from build123d import *

# Parameters (mm, degrees)
SKETCH1_R           = 8.5
BOSS_EXTRUDE1_DEPTH = 1
SKETCH2_W           = 31
SKETCH2_H           = 23.6
BOSS_EXTRUDE2_DEPTH = 4
SKETCH3_W           = 10
SKETCH3_H           = 23.6
BOSS_EXTRUDE3_DEPTH = 6
SKETCH4_R           = 3.5
BOSS_EXTRUDE4_DEPTH = 1
SKETCH5_R           = 2.5
BOSS_EXTRUDE5_DEPTH = 20.25
SKETCH7_R           = 2.25
CUT_EXTRUDE1_DEPTH  = 12
SKETCH8_R           = 2.25
CUT_EXTRUDE2_DEPTH  = 50.945194964
CHAMFER1_SIZE       = 0.5


with BuildPart() as part:
    # Sketch1 → Boss-Extrude1 (new body)
    with BuildSketch(Plane.XY):
        with Locations((15.5, 11.8)):
            Circle(SKETCH1_R)
    extrude(amount=BOSS_EXTRUDE1_DEPTH)

    # Sketch2 → Boss-Extrude2 (add)
    with BuildSketch(Plane.XY.offset(1)):
        with Locations((15.5, 11.8)):
            Rectangle(SKETCH2_W, SKETCH2_H)
    extrude(amount=BOSS_EXTRUDE2_DEPTH)

    # Sketch3 → Boss-Extrude3 (add)
    with BuildSketch(Plane.XY.offset(5)):
        with Locations((15.5, 11.8)):
            Rectangle(SKETCH3_W, SKETCH3_H)
    extrude(amount=BOSS_EXTRUDE3_DEPTH)

    # Sketch4 → Boss-Extrude4 (add)
    with BuildSketch(Plane.XY.offset(11)):
        with Locations((15.5, 11.8)):
            Circle(SKETCH4_R)
    extrude(amount=BOSS_EXTRUDE4_DEPTH)

    # Sketch5 → Boss-Extrude5 (add)
    with BuildSketch(Plane.XY.offset(12)):
        with Locations((15.5, 11.8)):
            Circle(SKETCH5_R)
    extrude(amount=BOSS_EXTRUDE5_DEPTH)

    # Sketch7 → Cut-Extrude1 (cut)
    with BuildSketch(Plane.XY.offset(32.25)):
        with Locations((15.5, 11.8)):
            Circle(SKETCH7_R)
    extrude(amount=-CUT_EXTRUDE1_DEPTH, mode=Mode.SUBTRACT)

    # Sketch8 → Cut-Extrude2 (cut, through all)
    with BuildSketch(Plane(origin=(0, 0, 1), x_dir=(-1, 0, 0), z_dir=(0, 0, -1))):
        with Locations((-26.5, 4.3)):
            Circle(SKETCH8_R)
        with Locations((-4.5, 19.3)):
            Circle(SKETCH8_R)
    extrude(amount=-CUT_EXTRUDE2_DEPTH, mode=Mode.SUBTRACT)

    # Chamfer1
    # the kernel refuses this chamfer: 0.5 mm, written as the material it takes off along each edge
    with BuildSketch(Plane(origin=(15.5, 11.8, 32.25), x_dir=(1, 0, 0), z_dir=(0, -1, 0))) as chamfer1_piece_1:
        Polygon((2.5, -CHAMFER1_SIZE), (2.5 - CHAMFER1_SIZE, 0), (2.5, 0), align=None)
    revolve(axis=Axis((15.5, 11.8, 32.25), (0, 0, 1)), mode=Mode.SUBTRACT)


solid = part.part
The listing builds one solid part. Answer for the finished solid, in the listing's coordinates (mm). A direction names the side the tool comes from. Coordinates: 2 decimals unless noted, no trailing zeros. Loops run counter-clockwise (first coordinate to the right, second up) from the corner with the lowest first, then second, coordinate; pieces in that order, holes last. Notation, with made-up numbers: (14, 11) -> (24, 11) arc R27 ccw to (24, 29) -> close; hole circle Ø4 at (67, 58.25). An arc over 180 degrees is marked (long way). Write item = value, one per line. Start each with the question number.
1) A cutting plane is placed at A-A (y = 4.3). Give the vertices of the cut face in (x, z), then the cut area to 3 significant figures.
2) A tool of negligible diameter and unlimited length cuts with its end or side. For faces 4 (the face through (0, 12, 3)), 5 (the face through (26, 12, 5)), 6 (the face through (5, 12, 5)), 7 (the face through (12, 20, 1)), 8 (the face through (17.646, 12.476, 26.207)), from which of +Z, -Z, +X, -X, +Y, -Y can it reach the whole face along a straight path? Write none if from no direction.
3) Straight lines are drawn through the part: line 1 (Y direction, x = 15.5, z = 28); line 2 (Z direction, x = 4.5, y = 11.5); line 3 (X direction, y = 12, z = 27.5). For each, find the intervals that lie inside material, in ascending order. Write a range as from..to.
4) A cutting plane is placed at B-B (x = 4.5). Give the vertices of the cut face in (y, z).
5) Given pin 1 Ø2 at (x, y) = (5.5, 18.5) entering from +Z; pin 2 Ø3 at (y, z) = (10, 8) entering from -X; pin 3 Ø4 at (y, z) = (17.5, 25) entering from -X; pin 4 Ø5 at (x, y) = (20, 20.5) entering from +Z, each flat-ended and moving along its own axis, determine where each tip first touches the part or whether it passes through.
6) A cutting plane is placed at D-D (x = 15.5). Give the vertices of the cut face in (y, z), then the cut area to 3 significant figures.
7) The mould has two halves that part along Y. Classify faces 1 (the face through (15, 0, 5)), 2 (the face through (24.354, 4.976, 2.972)), 3 (the face through (13, 13, 12)): released by +Y, released by -Y, zero draft, split by the parting line, or undercut.
8) A cutting plane is placed at C-C (y = 11.8). Give the vertices of the cut face in (x, z), then the cut area to 3 significant figures.
Responses:
q1.outline = (0, 1) -> (11.5, 1) -> (11.5, 0) -> (19.5, 0) -> (19.5, 1) -> (24.25, 1) -> (24.25, 5) -> (20.5, 5) -> (20.5, 11) -> (10.5, 11) -> (10.5, 5) -> (0, 5) -> close; (28.75, 1) -> (31, 1) -> (31, 5) -> (28.75, 5) -> close
q1.area = 174 mm²
q2.face_4 = +Z, -Z, -X, +Y, -Y
q2.face_5 = +Z, +X, +Y, -Y
q2.face_6 = +Z, -X, +Y, -Y
q2.face_7 = -Z
q2.face_8 = +Z
q3.line_1 = 9.3..9.55, 14.05..14.3
q3.line_2 = 1..5
q3.line_3 = 13.01..13.26, 17.74..17.99
q4.outline = (0, 1) -> (17.05, 1) -> (17.05, 5) -> (0, 5) -> close; (21.55, 1) -> (23.6, 1) -> (23.6, 5) -> (21.55, 5) -> close
q5.pin_1 = 5
q5.pin_2 = 10.5
q5.pin_3 = through
q5.pin_4 = 11
q6.outline = (0, 1) -> (3.3, 1) -> (3.3, 0) -> (20.3, 0) -> (20.3, 1) -> (23.6, 1) -> (23.6, 11) -> (15.3, 11) -> (15.3, 12) -> (14.3, 12) -> (14.3, 31.75) -> (14.05, 32) -> (14.05, 20.25) -> (9.55, 20.25) -> (9.55, 32) -> (9.3, 31.75) -> (9.3, 12) -> (8.3, 12) -> (8.3, 11) -> (0, 11) -> close
q6.area = 307 mm²
q7.face_1 = released by -Y
q7.face_2 = undercut
q7.face_3 = zero draft
q8.outline = (0, 1) -> (7, 1) -> (7, 0) -> (24, 0) -> (24, 1) -> (31, 1) -> (31, 5) -> (20.5, 5) -> (20.5, 11) -> (19, 11) -> (19, 12) -> (18, 12) -> (18, 31.75) -> (17.75, 32) -> (17.75, 20.25) -> (13.25, 20.25) -> (13.25, 32) -> (13, 31.75) -> (13, 12) -> (12, 12) -> (12, 11) -> (10.5, 11) -> (10.5, 5) -> (0, 5) -> close
q8.area = 255 mm²
